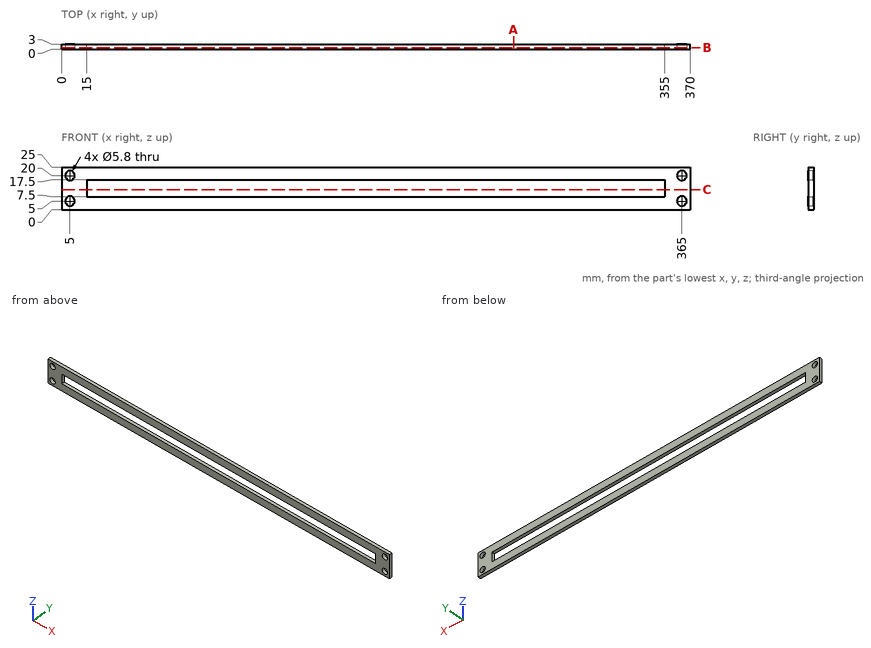
The figure shows three views and two pictorial views of one solid part (mm, origin at its lowest corner). Answer the questions. Coordinates: 2 decimals unless noted, no trailing zeros. Loops run counter-clockwise (first coordinate to the right, second up) from the corner with the lowest first, then second, coordinate; pieces in that order, holes last. Notation, with made-up numbers: (41.5, -3.5) -> (95.5, -3.5) arc R28 cw to (95.5, 32.5) -> close; hole circle Ø8 at (69.25, 74). An arc over 180 degrees is marked (long way). Write item = value, one per line. Start each with the question number.
1) A cutting plane is placed at C-C (z = 11.75). Give the vertices of the cut face in (x, y), then the cut area to 3 significant figures.
2) A cutting plane is placed at B-B (y = 0.8). Give the vertices of the cut face in (x, z).
3) Given pin 1 Ø3.5 at (x, z) = (365, 5) entering from +Y, flat-ended and moving along its own axis, determine where the tip first touches the part or whether it passes through.
4) A cutting plane is placed at A-A (x = 266). Give the vertices of the cut face in (y, z), then the cut area to 3 significant figures.
5) Straight lines are drawn through the part: line 1 (Z direction, x = 5, y = 1.25); line 2 (X direction, y = 0.8, z = 4.75); line 3 (Z direction, x = 46, y = 1.4). For each, find the intervals that lie inside material, in ascending order. Write a range as from..to.
Responses:
q1.outline = (0, 0) -> (15, 0) -> (15, 3) -> (0, 3) -> close; (355, 0) -> (370, 0) -> (370, 3) -> (355, 3) -> close
q1.area = 90.0 mm²
q2.outline = (0, 0) -> (370, 0) -> (370, 25) -> (0, 25) -> close; hole circle Ø5.8 at (5, 5); hole circle Ø5.8 at (5, 20); hole (15, 7.5) -> (355, 7.5) -> (355, 17.5) -> (15, 17.5) -> close; hole circle Ø5.8 at (365, 5); hole circle Ø5.8 at (365, 20)
q3.pin_1 = through
q4.outline = (0, 0) -> (3, 0) -> (3, 7.5) -> (0, 7.5) -> close; (0, 17.5) -> (3, 17.5) -> (3, 25) -> (0, 25) -> close
q4.area = 45.0 mm²
q5.line_1 = 0..2.1, 7.9..17.1, 22.9..25
q5.line_2 = 0..2.11, 7.89..362.11, 367.89..370
q5.line_3 = 0..7.5, 17.5..25
